Check sheet for the modelled part. Datum: model origin and axes. Units: mm. Face numbers are marked on the shaded views. A direction names the side the tool comes from. Coordinates: 2 decimals unless noted, no trailing zeros. Write each loop counter-clockwise with the first axis right and the second up, starting at its lowest first coordinate (ties: lowest second). Pieces come first, ordered by that corner, then holes. Notation, with made-up numbers: M 78.5,12 L 125.5,12 A7 ccw 125.5,21 Z; hole C 65,59 d4. An arc over 180 degrees is marked long. Answer as CSV lines item,"result". Start each with the question number.
Q1. Access from +Z, -Z, +X, -X, +Y, -Y to the whole of each face (thin tool, end or side, straight path). Record for the marked faces 5 and 6.
Q2. Sectioned sample at D-D, the plane y = 335. Record the cut outline in (x, z), then the cut area to 3 significant figures.
Q3. Sectioned sample at A-A, the plane x = 0. Record the cut outline in (y, z), then the cut area to 3 significant figures.
Q4. Thickness scan on line 1 along Y through (x, z) = (8, -24.45); line 2 along Z through (x, y) = (19.5, 289.5); line 3 along Y through (x, z) = (0, -24.6). Record the ranges inside material, lowest first. Write a range as from..to.
Q5. Depth check by flat-ended pin: pin 1 Ø2.5 at (x, y) = (15, 385) entering from -Z; pin 2 Ø6.5 at (x, y) = (15, 385) entering from -Z. Enter the tip coordinate at first touch or a pass-through.
Q6. Sectioned sample at B-B, the plane y = 15. Record the cut outline in (x, z).
Q7. Sectioned sample at C-C, the plane z = 3.5. Record the cut outline in (x, y), then the cut area to 3 significant figures.
Q8. Mould release check, pull along X, two halves, no side actions. Record for the marked faces 1, 2, 3 and 4: pulls with the +X half, pulls with the -X half, needs draft (parallel to the pull), parting line crosses it, or undercut.
Autodesk Inventor part; units mm, degrees
ref_plane "YZ Plane" through (0, 0, 0) normal (1, 0, 0) x (0, 1, 0)
ref_plane "XZ Plane" through (0, 0, 0) normal (0, 1, 0) x (-1, 0, 0)
ref_plane "XY Plane" through (0, 0, 0) normal (0, 0, 1) x (1, 0, 0)
sketch "Sketch1" plane through (0, 0, 0) normal (0, 1, 0) x (-1, 0, 0)
  line L0 (25, 25) -> (-25, 25)
  line L1 (-25, 25) -> (-25, -25)
  line L2 (-25, -25) -> (25, -25)
  line L3 (25, -25) -> (25, 25)
  line L4 (25, 25) -> (-25, -25) construction
  line L5 (-25, 25) -> (25, -25) construction
  line L6 (24, 24) -> (-24, 24)
  line L7 (-24, 24) -> (-24, -24)
  line L8 (-24, -24) -> (24, -24)
  line L9 (24, -24) -> (24, 24)
  line L10 (24, 24) -> (-24, -24) construction
  line L11 (-24, 24) -> (24, -24) construction
  point P0 (0, 0)
  dimension "d0" = 50
  dimension "d2" = 48
extrude "Extrusion1" add sketch "Sketch1" along normal blind 400
sketch "Sketch3" plane through (25, 0, -25) normal (0, 0, -1) x (-1, 0, 0)
  line L0 (50, 0) -> (50, 400)
  line L1 (0, 0) -> (50, 0)
  line L2 (50, 0) -> (50, 30)
  line L3 (50, 30) -> (0, 30)
  line L4 (0, 30) -> (0, 0)
  line L5 (50, 30) -> (0, 0) construction
  line L6 (0, 0) -> (0, 400)
  line L7 (50, 0) -> (50, 400)
  line L8 (0, 400) -> (50, 400)
  line L9 (50, 400) -> (50, 370)
  line L10 (50, 370) -> (0, 370)
  line L11 (0, 370) -> (0, 400)
  line L12 (0, 400) -> (50, 370) construction
  circle A0 centre (40, 385) radius 2
  line L13 (25, 385) -> (40, 385) construction
  line L14 (25, 385) -> (10, 385) construction
  circle A1 centre (10, 385) radius 2
  circle A2 centre (25, 15) radius 3.5
  line L15 (17, 23) -> (33, 23) construction
  line L16 (33, 23) -> (33, 7) construction
  line L17 (33, 7) -> (17, 7) construction
  line L18 (17, 7) -> (17, 23) construction
  line L19 (17, 23) -> (33, 7) construction
  line L20 (33, 23) -> (17, 7) construction
  circle A3 centre (17, 23) radius 2
  circle A4 centre (33, 23) radius 2
  circle A5 centre (33, 7) radius 2
  circle A6 centre (17, 7) radius 2
  line L21 (25, 15) -> (29.6644, 19.6644) construction
  point P0 (25, 0)
  dimension "d19" = 30
  dimension "d28" = 30
  dimension "d29" = 4
  dimension "d30" = 15
  dimension "d31" = 15
  dimension "d32" = 4
  dimension "d33" = 7
  dimension "d34" = 16
  dimension "d35" = 4
extrude "Extrusion3" cut sketch "Sketch3" against normal blind 50 contours A0 | A1 | A2 | A3 | A4 | A5 | A6
sketch "Sketch4" plane through (25, 0, 25) normal (1, 0, 0) x (0, 0, -1)
  line L0 (50, 0) -> (0, 0) construction
  line L1 (0, 0) -> (10.1, 0) construction
  line L2 (10.1, 0) -> (40.1, 0)
  line L3 (40.1, 0) -> (40.1, 20)
  line L4 (40.1, 20) -> (10.1, 20)
  line L5 (10.1, 20) -> (10.1, 0)
  point P0 (25, 0)
  dimension "d23" = 10.1
  dimension "d24" = 30
  dimension "d25" = 20
extrude "Extrusion4" cut sketch "Sketch4" against normal blind 10
properties part number "End-Link" material "Aluminum 6061"
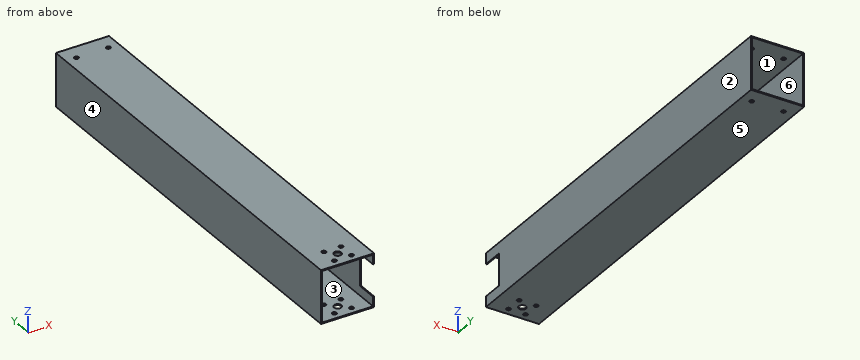
Output:
1,face 5,"-Z, +X, -X, +Y, -Y"
1,face 6,"+Y, -Y"
2,outline,"M -25,-25 L 25,-25 L 25,25 L -25,25 Z; hole M -24,-24 L 24,-24 L 24,24 L -24,24 Z"
2,area,"196 mm^2"
3,outline,"M 0,-25 L 11.5,-25 L 11.5,-24 L 0,-24 Z; M 0,24 L 11.5,24 L 11.5,25 L 0,25 Z; M 18.5,-25 L 400,-25 L 400,-24 L 18.5,-24 Z; M 18.5,24 L 400,24 L 400,25 L 18.5,25 Z"
3,area,"786 mm^2"
4,line 1,"y = 0..5, 9..21, 25..400"
4,line 2,"z = -25..-24, 24..25"
4,line 3,"y = 0..11.5, 18.5..400"
5,pin 1,"passes through"
5,pin 2,"stops at z = -25"
6,outline,"M -25,-25 L -3.5,-25 L -3.5,-24 L -24,-24 L -24,24 L -3.5,24 L -3.5,25 L -25,25 Z; M 3.5,-25 L 25,-25 L 25,-15.1 L 24,-15.1 L 24,-24 L 3.5,-24 Z; M 3.5,24 L 24,24 L 24,14.9 L 25,14.9 L 25,25 L 3.5,25 Z"
7,outline,"M -25,0 L -24,0 L -24,400 L -25,400 Z; M 24,20 L 25,20 L 25,400 L 24,400 Z"
7,area,"780 mm^2"
8,face 1,"undercut"
8,face 2,"pulls with the +X half"
8,face 3,"undercut"
8,face 4,"pulls with the -X half"
